Build history of the part. All positions in model axes, mm. Face numbers are marked on the shaded views. A direction names the side the tool comes from. Give positions to 0.01 mm unless a question says otherwise; leave off trailing zeros. Loops run counter-clockwise (first coordinate to the right, second up) from the corner with the lowest first, then second, coordinate; pieces in that order, holes last.
1) Two-plate mould, pull along Z, no slides. Class the marked faces 3, 4 and 5: +Z half, -Z half, draft (parallel to the pull), parting line (faces both ways), or undercut.
2) Band-saw the part on B-B on x = 2.25. List the corners of the cut face in (y, z), then the cut area to 3 significant figures.
3) Flat gauge pins, fed straight in: P1, Ø1.5, axis at y = -4, z = -4, coming from the +X side; P2, Ø11, axis at x = 5.5, z = -5.5, coming from the -Y side; P3, Ø1.1, axis at y = -6.5, z = -9.5, coming from the +X side; P4, Ø0.5, axis at x = 4.5, z = 9.5, coming from the -Y side. Where does each tip first touch, or does it go through?
4) Band-saw the part on C-C on z = 4.75. List the corners of the cut face in (x, y).
5) Wall check: line 1 (Y direction, x = 2.25, z = -0.5); line 2 (Z direction, x = 2.5, y = -7.5); line 3 (X direction, y = -4.5, z = -0.25). Give the ranges that are in metal, low to high.
6) 3-axis set-ups, long thin cutter, end or side, ignore diameter. For the marked faces 1 and 2: which of +Z, -Z, +X, -X, +Y, -Y reach the whole face in a straight line?
7) Band-saw the part on A-A on y = -2.75. List the corners of the cut face in (x, z).
8) Band-saw the part on D-D on z = 2. List the corners of the cut face in (x, y).
```python
from build123d import *

# Parameters (mm, degrees)
F0_W     = 20
F0_H     = 20
F1_DEPTH = 10
F3_DEPTH = 10
F4_DEPTH = 10
F6_DEPTH = 10


with BuildPart() as f1:
    # F0 (on Top) → F1 (new body)
    with BuildSketch(Plane.XY):
        Rectangle(F0_W, F0_H)
    extrude(amount=F1_DEPTH)

    # F2 (on face) → F3 (cut)
    with BuildSketch(Plane.YZ.offset(10)):
        Polygon((-9, 9), (-9, 10), (-10, 10), (-10, 0), (0, 0), align=None)
    extrude(amount=-F3_DEPTH, mode=Mode.SUBTRACT)

    # F0 (on Top) → F4 (join)
    with BuildSketch(Plane.XY):
        Rectangle(F0_W, F0_H)
    extrude(amount=-F4_DEPTH)

    # F5 (on face) → F6 (cut)
    with BuildSketch(Plane.XZ.offset(10)):
        Polygon((10, 0), (0, 0), (0, -1), (8, -9), (8, -10), (10, -10), align=None)
    extrude(amount=-F6_DEPTH, mode=Mode.SUBTRACT)


solid = f1.part
```
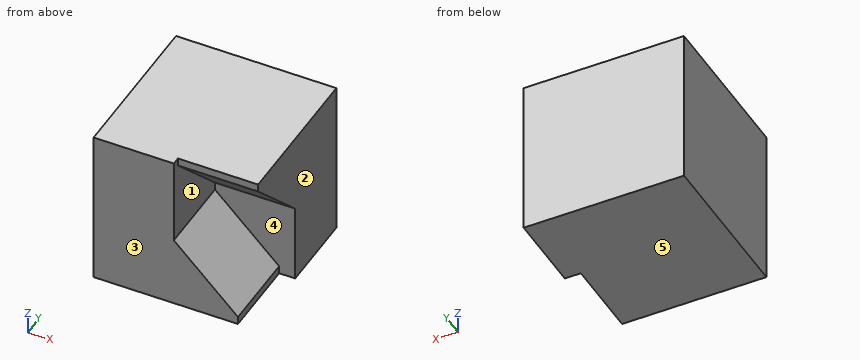
Findings below:
1. face 3: draft
1. face 4: undercut
1. face 5: -Z half
2. outline: (-10, -10) - (10, -10) - (10, 10) - (-9, 10) - (-9, 9) - (0, 0) - (0, -3.25) - (-10, -3.25) - close
2. area: 317 mm2
3. P1: stops at x = 3.75
3. P2: stops at y = -10
3. P3: stops at x = 8
3. P4: stops at y = -9
4. outline: (-10, -10) - (0, -10) - (0, -4.75) - (10, -4.75) - (10, 10) - (-10, 10) - close
5. line 1: y = 0 to 10
5. line 2: z = -10 to -3.5, 7.5 to 10
5. line 3: x = -10 to 0
6. face 1: +X, -Y
6. face 2: +Z, -Z, +X, +Y, -Y
7. outline: (-10, -10) - (8, -10) - (8, -9) - (0, -1) - (0, 2.75) - (10, 2.75) - (10, 10) - (-10, 10) - close
8. outline: (-10, -10) - (0, -10) - (0, -2) - (10, -2) - (10, 10) - (-10, 10) - close
